from build123d import *

# Parameters (mm, degrees)
SKETCH1_R               = 23.8
BOSS_EXTRUDE1_DEPTH     = 2.3
SKETCH2_R               = 23.8
SKETCH2_R_2             = 20.2
BOSS_EXTRUDE2_DEPTH     = 10
SKETCH3_R               = 3
BOSS_EXTRUDE3_DEPTH     = 9.7
CHAMFER1_SIZE           = 6
CHAMFER1_SIZE2          = 1.057961884
SKETCH4_R               = 1.25
CUT_EXTRUDE1_DEPTH      = 15
CUT_EXTRUDE3_START      = -9.2
SKETCH6_R               = 22.5
SKETCH6_R_2             = 20.2
CUT_EXTRUDE3_DEPTH      = 9.2
SKETCH7_R               = 1.5
CUT_EXTRUDE4_DEPTH      = 5
REDONDEO1_R             = 1.2
SALIENTE_EXTRUIR1_START = 1
CROQUIS1_R              = 9.339254136
CROQUIS1_R_2            = 1.25
SALIENTE_EXTRUIR1_DEPTH = 1
CROQUIS2_R              = 2
SALIENTE_EXTRUIR2_DEPTH = 3


with BuildPart() as part:
    # Sketch1 → Boss-Extrude1 (new body)
    with BuildSketch(Plane.XY):
        Circle(SKETCH1_R)
    extrude(amount=BOSS_EXTRUDE1_DEPTH)

    # Sketch2 → Boss-Extrude2 (add)
    with BuildSketch(Plane.XY.offset(2.3)):
        Circle(SKETCH2_R)
        Circle(SKETCH2_R_2, mode=Mode.SUBTRACT)
    extrude(amount=BOSS_EXTRUDE2_DEPTH)

    # Sketch3 → Boss-Extrude3 (add)
    with BuildSketch(Plane.XY.offset(2.3)):
        Circle(SKETCH3_R)
    extrude(amount=BOSS_EXTRUDE3_DEPTH)

    # Chamfer1
    chamfer1_edges = [part.edges().sort_by_distance(p)[0] for p in [
        (-23.8, 0, 0),
    ]]
    chamfer1_side = [part.faces().sort_by_distance(p)[0] for p in [
        (0, 0, 0),
    ]]
    chamfer(chamfer1_edges, length=CHAMFER1_SIZE, length2=CHAMFER1_SIZE2, reference=chamfer1_side[0])

    # Sketch4 → Cut-Extrude1 (cut)
    with BuildSketch(Plane(origin=(0, 0, 0), x_dir=(-1, 0, 0), z_dir=(0, 0, -1))):
        with Locations((6, 0)):
            Circle(SKETCH4_R)
        with Locations((0, -6)):
            Circle(SKETCH4_R)
        with Locations((-6, 0)):
            Circle(SKETCH4_R)
        with Locations((0, 6)):
            Circle(SKETCH4_R)
    extrude(amount=-CUT_EXTRUDE1_DEPTH, mode=Mode.SUBTRACT)

    # Sketch6 → Cut-Extrude3 (cut)
    with BuildSketch(Plane.XY.offset(12.3).offset(CUT_EXTRUDE3_START)):
        Circle(SKETCH6_R)
        Circle(SKETCH6_R_2, mode=Mode.SUBTRACT)
    extrude(amount=CUT_EXTRUDE3_DEPTH, mode=Mode.SUBTRACT)

    # Sketch7 → Cut-Extrude4 (cut)
    with BuildSketch(Plane.XY.offset(12)):
        Circle(SKETCH7_R)
    extrude(amount=-CUT_EXTRUDE4_DEPTH, mode=Mode.SUBTRACT)

    # Redondeo1
    redondeo1_edges = [part.edges().sort_by_distance(p)[0] for p in [
        (-3, 0, 2.3),
    ]]
    fillet(redondeo1_edges, radius=REDONDEO1_R)

    # Croquis1 → Saliente-Extruir1 (add)
    with BuildSketch(Plane(origin=(0, 0, 0), x_dir=(-1, 0, 0), z_dir=(0, 0, -1)).offset(SALIENTE_EXTRUIR1_START)):
        Circle(CROQUIS1_R)
        with Locations((0, 6)):
            Circle(CROQUIS1_R_2, mode=Mode.SUBTRACT)
        with Locations((6, 0)):
            Circle(CROQUIS1_R_2, mode=Mode.SUBTRACT)
        with Locations((0, -6)):
            Circle(CROQUIS1_R_2, mode=Mode.SUBTRACT)
        with Locations((-6, 0)):
            Circle(CROQUIS1_R_2, mode=Mode.SUBTRACT)
    extrude(amount=-SALIENTE_EXTRUIR1_DEPTH)

    # Croquis2 → Saliente-Extruir2 (add)
    with BuildSketch(Plane(origin=(0, 0, -1), x_dir=(-1, 0, 0), z_dir=(0, 0, -1))):
        Circle(CROQUIS2_R)
    extrude(amount=SALIENTE_EXTRUIR2_DEPTH)


solid = part.part
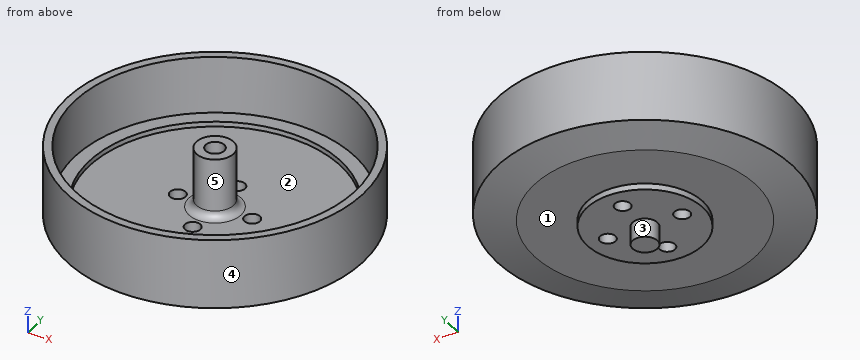
Source: CAD feature listing. Evaluate the final solid. Frame: model axes, mm. Face numbers are marked on the shaded views. A direction names the side the tool comes from. Round coordinates to 2 decimals unless told otherwise and drop trailing zeros. Loops run counter-clockwise (first coordinate to the right, second up) from the corner with the lowest first, then second, coordinate; pieces in that order, holes last. Notation, with made-up numbers: M 50,32.25 L 69,32.25 A12 ccw 69,37.25 Z; hole C 2,50 d4. An arc over 180 degrees is marked long. Return JSON: item names as keys, results as strings. Group by question number.
1. Pin query (flat end, axial travel): pin 1 (2.5 mm diameter, centred on x = 0, y = 0, fed in from +Z); pin 2 (3 mm diameter, centred on x = 0, y = -6, fed in from -Z); pin 3 (3.5 mm diameter, centred on x = 0, y = -0.5, fed in from +Z). Return the tip coordinate at first contact, or that it passes through.
2. Material intervals for line 1 along Y through (x, z) = (0, 1.4); line 2 along Y through (x, z) = (0, -0.1); line 3 along X through (y, z) = (1, 6.5), sorted ascending. Write a range as from..to.
3. Section query B-B on x = 0. State how many separate pieces and enclosed holes the cut face has, and give its area (3 significant figures).
4. Mould query, pull axis X, two halves, no side actions, for the marked faces 1, 2 and 3. Classes: released by +X, released by -X, zero draft, split by the parting line, or undercut.
5. Reachability of the marked faces 4 and 5 from +Z, -Z, +X, -X, +Y, -Y: full face, straight path, thin tool, end or side. Return the list, or none.
6. Section query A-A on z = 9.25. Output: boundary loops of the cut face in (x, y).
Checks:
{
 "1": {"pin 1": "stops at z = 7", "pin 2": "stops at z = -1", "pin 3": "stops at z = 12"},
 "2": {"line 1": "y = -23.8..-7.25, -4.75..4.75, 7.25..23.8", "line 2": "y = -9.34..-7.25, -4.75..4.75, 7.25..9.34", "line 3": "x = -23.78..-22.48, -2.83..2.83, 22.48..23.78"},
 "3": {"separate pieces": "3", "enclosed holes": "0", "area": "191 mm²"},
 "4": {"face 1": "zero draft", "face 2": "undercut", "face 3": "split by the parting line"},
 "5": {"face 4": "+Z, -Z", "face 5": "+Z"},
 "6": {"outline": "C 0,0 d47.6; C 0,0 d6; hole C 0,0 d45; hole C 0,0 d3"}
}
